Check sheet for the modelled part. Datum: model origin and axes. Units: mm. Face numbers are marked on the shaded views. Coordinates: 2 decimals unless noted, no trailing zeros. Write each loop counter-clockwise with the first axis right and the second up, starting at its lowest first coordinate (ties: lowest second). Pieces come first, ordered by that corner, then holes. Notation, with made-up numbers: (12.5, -17) -> (41.5, -17) arc R22 cw to (41.5, 15) -> close; hole circle Ø2 at (25, -37). An arc over 180 degrees is marked (long way). One line per item, written item: value. Start each with the question number.
1) Sectioned sample at A-A on z = -42.5. Enter the section's corners in (x, y).
2) Gauge pin test, flat ends, axial feed: P1, Ø0.6, axis at x = -68, y = 13.5, coming from the -Z side; P2, Ø0.6, axis at x = 68, y = 13.5, coming from the +Z side; P3, Ø10, axis at x = 53.5, z = 16.5, coming from the +Y side. Record the tip position at first contact, or that the pin passes through.
3) Sectioned sample at D-D on y = 10. Give the number of separate pieces and of enclosed holes in the cut face, plus the area to 3 significant figures.
4) Sectioned sample at C-C on x = 0. Enter the section's corners in (y, z).
5) Draft check along X on the marked faces 1, 2 and 3. Enter one of: +X half, -X half, draft (parallel to the pull), parting line (faces both ways), or undercut.
6) Scan lines: line 1 along X through (y, z) = (11, -42.5); line 2 along X through (y, z) = (7.5, -18.5); line 3 along Z through (x, y) = (26, 8.25). Record each from-to range of solid material in increasing order. Write a range as [from, to].
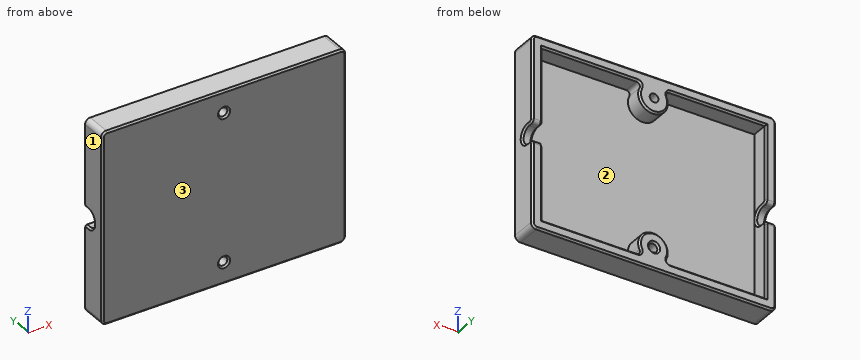
```python
from build123d import *

# Parameters (mm, degrees)
SKETCH1_W           = 140
SKETCH1_H           = 110
BOSS_EXTRUDE1_DEPTH = 16
SKETCH2_R           = 2.5
CUT_EXTRUDE1_DEPTH  = 91.44888059
FILLET1_R           = 3
SHELL1_T            = -6
CUT_EXTRUDE2_DEPTH  = 152.26466871
FILLET2_R           = 2
CHAMFER2_SIZE       = 1


with BuildPart() as part:
    # Sketch1 → Boss-Extrude1 (new body)
    with BuildSketch(Plane(origin=(0, 0, 0), x_dir=(1, 0, 0), z_dir=(0, 1, 0))):
        Rectangle(SKETCH1_W, SKETCH1_H)
    extrude(amount=BOSS_EXTRUDE1_DEPTH)

    # Sketch2 → Cut-Extrude1 (cut, through all)
    with BuildSketch(Plane(origin=(0, 16, 0), x_dir=(1, 0, 0), z_dir=(0, 1, 0))):
        with Locations(Location((0, 42.5, 0), (0, 0, 270))):
            Circle(SKETCH2_R)
        with Locations(Location((0, -42.5, 0), (0, 0, 90))):
            Circle(SKETCH2_R)
    extrude(amount=-CUT_EXTRUDE1_DEPTH, mode=Mode.SUBTRACT)

    # Fillet1
    fillet1_edges = [part.edges().sort_by_distance(p)[0] for p in [
        (70, 8, 55),
        (-70, 8, 55),
        (-70, 8, -55),
        (70, 8, -55),
    ]]
    fillet(fillet1_edges, radius=FILLET1_R)

    # Shell1
    shell1_openings = [part.faces().sort_by_distance(p)[0] for p in [
        (0, 16, 0),
    ]]
    offset(amount=SHELL1_T, openings=shell1_openings, kind=Kind.INTERSECTION)

    # Sketch3 → Cut-Extrude2 (cut, through all)
    with BuildSketch(Plane(origin=(70, 0, 0), x_dir=(0, 0, -1), z_dir=(1, 0, 0))):
        with BuildLine():
            Line((5, 20), (5, 12))
            ThreePointArc((5, 12), (0, 7), (-5, 12))
            Line((-5, 12), (-5, 20))
            ThreePointArc((-5, 20), (0, 25), (5, 20))
        make_face()
    extrude(amount=-CUT_EXTRUDE2_DEPTH, mode=Mode.SUBTRACT)

    # Fillet2
    fillet2_edges = [part.edges().sort_by_distance(p)[0] for p in [
        (-5.477225575, 11, -49),
        (5.477225575, 11, 49),
        (-5.477225575, 11, 49),
        (5.477225575, 11, -49),
        (67, 16, -5),
        (-67, 16, -5),
        (67, 16, 5),
        (-67, 16, 5),
    ]]
    fillet(fillet2_edges, radius=FILLET2_R)

    # Chamfer2
    chamfer2_edges = [part.edges().sort_by_distance(p)[0] for p in [
        (64, 13, -5),
        (64, 16, -28),
        (64, 15.414213562, -5.585786438),
        (64, 15.414213562, 5.585786438),
        (70, 13, 5),
        (70, 16, -29.5),
        (70, 15.414213562, -5.585786438),
        (70, 15.414213562, 5.585786438),
        (-36.74341649, 16, -49),
        (0, 16, -34),
        (-64, 13, 5),
        (-64, 15.414213562, 5.585786438),
        (-64, 15.414213562, -5.585786438),
        (-70, 13, 5),
        (-70, 15.414213562, 5.585786438),
        (-70, 15.414213562, -5.585786438),
        (-7.796524471, 16, 48.069044968),
        (7.796524471, 16, 48.069044968),
        (7.796524471, 16, -48.069044968),
        (-7.796524471, 16, -48.069044968),
        (0, 0, -45),
        (0, 16, -45),
        (0, 0, 45),
        (-70, 0, 0),
        (-70, 16, -29.5),
        (70, 0, 0),
        (0, 0, 55),
        (0, 0, -55),
        (69.121320344, 0, 54.121320344),
        (-69.121320344, 0, 54.121320344),
        (69.121320344, 0, -54.121320344),
        (-69.121320344, 0, -54.121320344),
        (0, 16, -55),
        (70, 16, 29.5),
        (0, 16, 55),
        (69.121320344, 16, 54.121320344),
        (-69.121320344, 16, 54.121320344),
        (69.121320344, 16, -54.121320344),
        (-69.121320344, 16, -54.121320344),
        (36.74341649, 16, -49),
        (-64, 16, -28),
        (-36.74341649, 16, 49),
        (64, 16, 28),
        (-64, 7, 0),
        (-64, 13, -5),
        (70, 13, -5),
        (70, 7, 0),
        (-70, 13, -5),
        (64, 7, 0),
        (-70, 7, 0),
        (64, 13, 5),
        (36.74341649, 16, 49),
        (0, 16, 34),
        (-64, 16, 28),
        (-70, 16, 29.5),
    ]]
    chamfer(chamfer2_edges, length=CHAMFER2_SIZE - 0.0001)  # a hair under: the kernel refuses the full size


solid = part.part
```
Answers:
1. outline: (-70, 1) -> (-69, 0) -> (-3.5, 0) -> (-2.5, 1) -> (-2.5, 15) -> (-3.5, 16) -> (-7.5, 16) -> (-8.5, 15) -> (-8.5, 6) -> (-64, 6) -> (-64, 15) -> (-65, 16) -> (-69, 16) -> (-70, 15) -> close; (2.5, 1) -> (3.5, 0) -> (69, 0) -> (70, 1) -> (70, 15) -> (69, 16) -> (65, 16) -> (64, 15) -> (64, 6) -> (8.5, 6) -> (8.5, 15) -> (7.5, 16) -> (3.5, 16) -> (2.5, 15) -> close
2. P1: stops at z = -54.92
2. P2: stops at z = 54.92
2. P3: stops at y = 6
3. separate pieces: 2
3. enclosed holes: 2
3. area: 3,130 mm2
4. outline: (0, -54) -> (1, -55) -> (15, -55) -> (16, -54) -> (16, -46) -> (15, -45) -> (1, -45) -> (0, -46) -> close; (0, -39) -> (1, -40) -> (15, -40) -> (16, -39) -> (16, -35) -> (15, -34) -> (6, -34) -> (6, 34) -> (15, 34) -> (16, 35) -> (16, 40) -> (1, 40) -> (0, 39) -> close; (0, 46) -> (1, 45) -> (16, 45) -> (16, 54) -> (15, 55) -> (1, 55) -> (0, 54) -> close
5. face 1: -X half
5. face 2: undercut
5. face 3: draft
6. line 1: x = [-70, -64], [-8.5, -2.5], [2.5, 8.5], [64, 70]
6. line 2: x = [-70, -64], [64, 70]
6. line 3: z = [-55, -49], [49, 55]
